Source: CAD feature listing. Evaluate the final solid. Frame: model axes, mm. Round coordinates to 2 decimals unless told otherwise and drop trailing zeros. Write each loop counter-clockwise with the first axis right and the second up, starting at its lowest first coordinate (ties: lowest second). Pieces come first, ordered by that corner, then holes. Notation, with made-up numbers: (39, -4.75) -> (95, -4.75) arc R15 cw to (95, 14.25) -> close; hole circle Ø5 at (-12.5, -31). An arc over 180 degrees is marked (long way). Put each result on its own line as item: value.
```python
from build123d import *

# Parameters (mm, degrees)
SKETCH1_R           = 5
BOSS_EXTRUDE1_DEPTH = 30


with BuildPart() as part:
    # Sketch1 → Boss-Extrude1 (new, symmetric)
    with BuildSketch(Plane(origin=(0, 0, 0), x_dir=(1, 0, 0), z_dir=(0, 1, 0))):
        with BuildLine():
            Line((0, -7), (25, -7))
            Line((25, -7), (25, -5))
            Line((25, -5), (4.898979486, -5))
            ThreePointArc((4.898979486, -5), (-2.645751311, 6.480740698), (0, -7))
        make_face()
        with Locations(Location((0, 0, 0), (0, 0, 270))):
            Circle(SKETCH1_R, mode=Mode.SUBTRACT)
    extrude(amount=BOSS_EXTRUDE1_DEPTH, both=True)


solid = part.part
```
Q1. Pin query (flat end, axial travel): pin 1 (1 mm diameter, centred on y = 18.5, z = 1.5, fed in from -X); pin 2 (4 mm diameter, centred on y = -18, z = 0, fed in from +X); pin 3 (6 mm diameter, centred on x = 8.5, y = 5, fed in from -Z). Return the tip coordinate at first contact, or that it passes through.
Ans:
pin 1: stops at x = -6.93
pin 2: stops at x = 7
pin 3: stops at z = -4.33
Q2. Draft query along X for faces 1 (the flat face through (25, 0, 6)), 2 (the flat face through (15, 0, 5)), 3 (the cylindrical face through (-4.88, -0.42, -1.08)). Return one class per face: +X half, -X half, draft (parallel to the pull), parting line (faces both ways), or undercut.
Ans:
face 1: +X half
face 2: draft
face 3: undercut
Q3. Cut plane D-D on x = 14.5. Output: boundary loops of the cut face in (y, z), and give its area (3 significant figures).
Ans:
outline: (-30, 5) -> (30, 5) -> (30, 7) -> (-30, 7) -> close
area: 120 mm^2
Q4. Cut plane C-C on x = -3.5. Output: boundary loops of the cut face in (y, z), and give its area (3 significant figures).
Ans:
outline: (-30, -6.06) -> (30, -6.06) -> (30, -3.57) -> (-30, -3.57) -> close; (-30, 3.57) -> (30, 3.57) -> (30, 6.06) -> (-30, 6.06) -> close
area: 299 mm^2
Q5. Cut plane A-A on z = 0. Output: boundary loops of the cut face in (x, y), and give its area (3 significant figures).
Ans:
outline: (-7, -30) -> (-5, -30) -> (-5, 30) -> (-7, 30) -> close; (5, -30) -> (7, -30) -> (7, 30) -> (5, 30) -> close
area: 240 mm^2
Q6. Cut plane B-B on y = -21.5. Output: boundary loops of the cut face in (x, z).
Ans:
outline: (0, 7) arc R7 ccw (long way) to (4.9, 5) -> (25, 5) -> (25, 7) -> close; hole circle Ø10 at (0, 0)
Q7. Material intervals for line 1 (X direction, y = -15, z = 0); line 2 (Z direction, x = 14.5, y = -27); line 3 (X direction, y = 4, z = -4), sorted ascending. Write a range as [from, to].
Ans:
line 1: x = [-7, -5], [5, 7]
line 2: z = [5, 7]
line 3: x = [-5.74, -3], [3, 5.74]
